Read the model definition and answer for the solid it produces. Units are mm, in the model's axes. Coordinates: 2 decimals unless noted, no trailing zeros. Loops run counter-clockwise (first coordinate to the right, second up) from the corner with the lowest first, then second, coordinate; pieces in that order, holes last. Notation, with made-up numbers: (52, 58.25) - (87, 58.25) arc R31 cw to (87, 87.25) - close; hole circle Ø6 at (30.5, 69.25). An arc over 180 degrees is marked (long way). One line per question, with ' | ' between items. Start each with the question number.
```python
from build123d import *

# Parameters (mm, degrees)
SKETCH1_W           = 218
SKETCH1_H           = 2
BOSS_EXTRUDE1_DEPTH = 298
SKETCH2_R           = 11
SKETCH2_R_2         = 1.5
CUT_EXTRUDE1_DEPTH  = 10


with BuildPart() as part:
    # Sketch1 → Boss-Extrude1 (new body)
    with BuildSketch(Plane(origin=(0, 0, 0), x_dir=(0, 0, -1), z_dir=(1, 0, 0))):
        with Locations((82.3216851, 1)):
            Rectangle(SKETCH1_W, SKETCH1_H)
    extrude(amount=BOSS_EXTRUDE1_DEPTH)

    # Sketch2 → Cut-Extrude1 (cut)
    with BuildSketch(Plane(origin=(0, 2, 0), x_dir=(1, 0, 0), z_dir=(0, 1, 0))):
        with Locations((74, 132.3216851)):
            Circle(SKETCH2_R)
        with Locations((89.5, 116.8216851)):
            Circle(SKETCH2_R_2)
        with Locations((58.5, 116.8216851)):
            Circle(SKETCH2_R_2)
        with Locations((89.5, 147.8216851)):
            Circle(SKETCH2_R_2)
        with Locations((58.5, 147.8216851)):
            Circle(SKETCH2_R_2)
        with Locations((256.33130124, 47.719426297)):
            Circle(SKETCH2_R_2)
        with Locations((256.457517214, 16.719426297)):
            Circle(SKETCH2_R_2)
        with Locations((225.33130124, 16.719426297)):
            Circle(SKETCH2_R_2)
        with Locations((225.33130124, 47.719426297)):
            Circle(SKETCH2_R_2)
        with Locations((240.957517214, 32.219426297)):
            Circle(SKETCH2_R)
        with Locations((290.5, 32.219426297)):
            Circle(SKETCH2_R_2)
        with Locations((7.5, 132.3216851)):
            Circle(SKETCH2_R_2)
        with Locations((207.490401532, 32.219426297)):
            Circle(SKETCH2_R_2)
        with Locations((207.490401532, 183.8216851)):
            Circle(SKETCH2_R_2)
        with Locations((207.490401532, -19.1783149)):
            Circle(SKETCH2_R_2)
        with Locations((7.5, -19.1783149)):
            Circle(SKETCH2_R_2)
        with Locations((7.5, 183.8216851)):
            Circle(SKETCH2_R_2)
        Polygon((15, 176.3216851), (57.721228679, 176.3216851), (57.721228679, 157.8216851), (51.65209525, 157.8216851), (51.65209525, 146.8216851), (15, 146.8216851), (15, 159.517007057), align=None)
        Polygon((149, -11.6783149), (104.471210326, -11.6783149), (15, -11.6783149), (15, 89.941809838), (15, 116.8216851), (49.873323929, 116.8216851), (49.873323929, 106.8216851), (99.5, 106.8216851), (99.5, 157.8216851), (87.721228679, 157.8216851), (87.721228679, 176.3216851), (101.200621078, 176.3216851), (149, 176.3216851), (283, 176.3216851), (283, 47.8216851), (263.876177895, 47.8216851), (263.876177895, 57.719426297), (214.790401532, 57.719426297), (214.790401532, 47.719426297), (199.990401532, 47.719426297), (199.990401532, 16.719426297), (214.790401532, 16.719426297), (214.790401532, 6.77711424), (226.154489119, 6.77711424), (226.154489119, -11.6783149), align=None)
        Polygon((283, -11.6783149), (283, 10.126363143), (283, 22.8216851), (263.305421964, 22.488619524), (263.305421964, 6.7816851), (256.695388827, 6.7816851), (256.695388827, -11.6783149), align=None)
    extrude(amount=-CUT_EXTRUDE1_DEPTH, mode=Mode.SUBTRACT)


solid = part.part
```
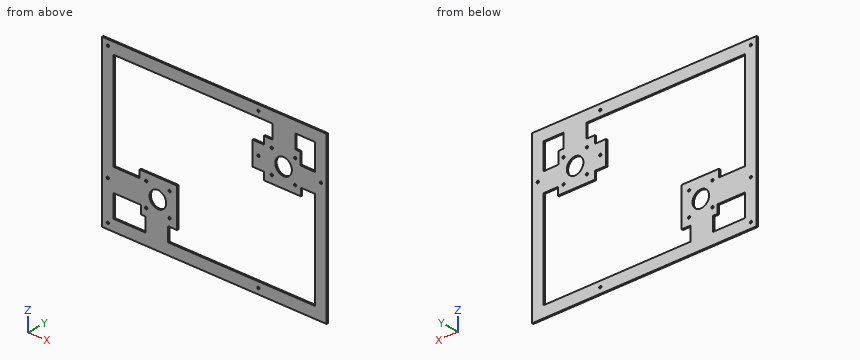
1) The part is cut by section B-B on x = 134.5. Write down the section's boundary in (y, z).
2) The part is cut by section C-C on x = 248. Write down the section's boundary in (y, z), and give its area (3 significant figures).
3) The part is cut by section D-D on y = 0.4. Count the separate pieces of the cut face and the enclosed holes in it, and give its area (3 significant figures).
4) The part is cut by section A-A on z = -111.5. Write down the section's boundary in (x, y), and give its area (3 significant figures).
5) Find the intervals of material crossed by line 1 along Z through (x, y) = (242, 1.45); line 2 along X through (y, z) = (1.4, 3.5); line 3 along Z through (x, y) = (279, 1.05), in increasing order. Write a range as from..to.
Answer below:
1) outline: (0, -191.32) - (2, -191.32) - (2, -176.32) - (0, -176.32) - close; (0, 11.68) - (2, 11.68) - (2, 26.68) - (0, 26.68) - close
2) outline: (0, -191.32) - (2, -191.32) - (2, -176.32) - (0, -176.32) - close; (0, -57.72) - (2, -57.72) - (2, -40.67) - (0, -40.67) - close; (0, -23.77) - (2, -23.77) - (2, 26.68) - (0, 26.68) - close | area: 165 mm2
3) separate pieces: 1 | enclosed holes: 20 | area: 21,800 mm2
4) outline: (0, 0) - (15, 0) - (15, 2) - (0, 2) - close; (49.87, 0) - (99.5, 0) - (99.5, 2) - (49.87, 2) - close; (283, 0) - (298, 0) - (298, 2) - (283, 2) - close | area: 159 mm2
5) line 1: -191.32..-176.32, -57.72..-43.17, -21.27..26.68 | line 2: 0..15, 226.15..256.7, 283..298 | line 3: -191.32..-176.32, -47.82..-22.75, 11.68..26.68
